Can you work these out from the model? Positions are in its coordinate system, mm. Round coordinates to 2 decimals unless told otherwise and drop trailing zeros. Order: outer loops, then holes, each group sorted by start corner. A loop starts at its lowest first (then second) coordinate and runs counter-clockwise, first axis right, second up.
Q1. If I drill on line 1 (X direction, y = 3.25, z = 36); line 2 (Z direction, x = 1, y = 3.25); line 3 (Z direction, x = -72.5, y = 3.25), over which ranges is the centre line in solid material (lowest first)?
Q2. If we section it at B-B (z = -36): Please give me the cut outline in (x, y).
Q3. If we section it at A-A (x = -32): Please give me the cut outline in (y, z), plus the area to 3 significant figures.
Q4. Will these pins go through, and if not, where does the flat tip stop? P1, Ø1.9, axis at y = 4, z = 59, coming from the -X side; P2, Ø1.9, axis at y = 2, z = -58.5, coming from the -X side; P3, Ø1.5, axis at x = -3.5, y = 3.5, coming from the -Z side; P4, Ø5.5, axis at x = 72.45, z = -59.75, coming from the +Y side.
Q5. If we section it at C-C (y = 5): Count the separate pieces of the cut face and the enclosed holes in it, plus the area to 3 significant figures.
from build123d import *

# Parameters (mm, degrees)
BOSS_EXTRUDE1_DEPTH     = 6.35
F_1_4_CLEARANCE_HOLE1_D = 7.14248


with BuildPart() as part:
    # Sketch1 → Boss-Extrude1 (new body)
    with BuildSketch(Plane(origin=(0, 0, 0), x_dir=(1, 0, 0), z_dir=(0, 1, 0))):
        Polygon((-88.9, -38.1), (-88.9, -57.15), (-69.85, -76.2), (-50.8, -76.2), (-50.8, -69.723), (50.8, -69.723), (50.8, -76.2), (69.85, -76.2), (88.9, -57.15), (88.9, -38.1), (82.423, -38.1), (82.423, 38.1), (88.9, 38.1), (88.9, 57.15), (69.85, 76.2), (50.8, 76.2), (50.8, 69.723), (-50.8, 69.723), (-50.8, 76.2), (-69.85, 76.2), (-88.9, 57.15), (-88.9, 38.1), (-82.423, 38.1), (-82.423, -38.1), align=None)
        Polygon((-57.15, -56.896), (-69.596, -44.45), (-69.596, -38.1), (-76.073, -38.1), (-76.073, 38.1), (-69.596, 38.1), (-69.596, 44.45), (-57.15, 56.896), (-50.8, 56.896), (-50.8, 63.373), (50.8, 63.373), (50.8, 56.896), (57.15, 56.896), (69.596, 44.45), (69.596, 38.1), (76.073, 38.1), (76.073, -38.1), (69.596, -38.1), (69.596, -44.45), (57.15, -56.896), (50.8, -56.896), (50.8, -63.373), (-50.8, -63.373), (-50.8, -56.896), align=None, mode=Mode.SUBTRACT)
    extrude(amount=BOSS_EXTRUDE1_DEPTH)

    # 1/4 Clearance Hole1 (through all)
    with Locations(Plane(origin=(0, 0, 0), x_dir=(-1, 0, 0), z_dir=(0, -1, 0))):
        with Locations((-72.452653333, 59.752653333), (72.452653333, 59.752653333), (72.452653333, -59.752653333), (-72.452653333, -59.752653333)):
            Hole(F_1_4_CLEARANCE_HOLE1_D / 2)


solid = part.part
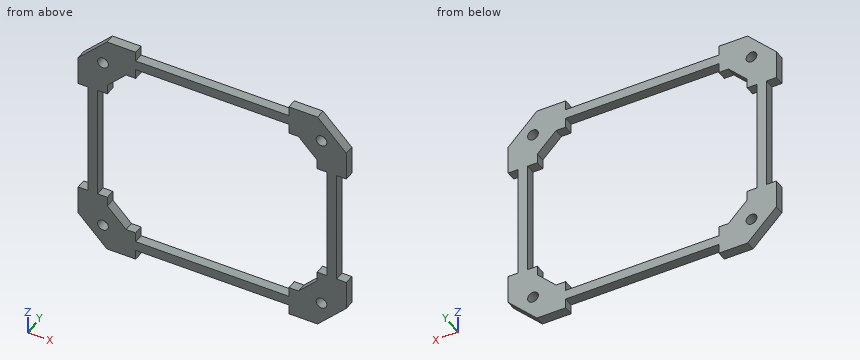
Solution:
1. line 1: x = -82.42 to -76.07, 76.07 to 82.42
1. line 2: z = -69.72 to -63.37, 63.37 to 69.72
1. line 3: z = -73.55 to -63.32, -56.18 to -38.1, 38.1 to 56.18, 63.32 to 73.55
2. outline: (-82.42, 0) - (-76.07, 0) - (-76.07, 6.35) - (-82.42, 6.35) - close; (76.07, 0) - (82.42, 0) - (82.42, 6.35) - (76.07, 6.35) - close
3. outline: (0, -69.72) - (6.35, -69.72) - (6.35, -63.37) - (0, -63.37) - close; (0, 63.37) - (6.35, 63.37) - (6.35, 69.72) - (0, 69.72) - close
3. area: 80.6 mm2
4. P1: stops at x = -88
4. P2: stops at x = -88.5
4. P3: stops at z = -69.72
4. P4: passes through
5. separate pieces: 1
5. enclosed holes: 5
5. area: 6,080 mm2
